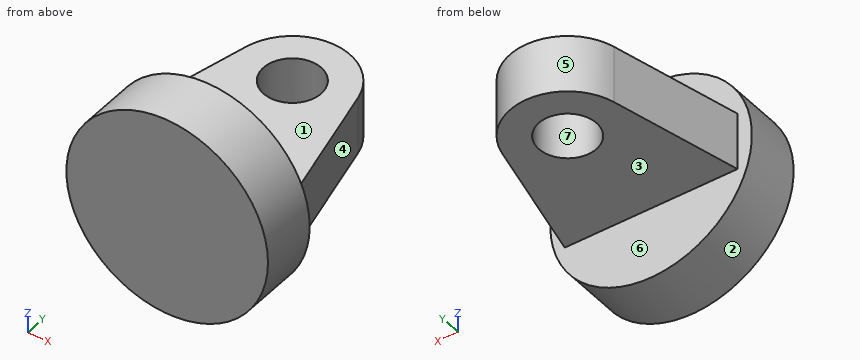
```python
from build123d import *

# Parameters (mm, degrees)
SKETCH_1_R           = 5
EXTRUDE_1_DEPTH      = 10
SKETCH_2_R           = 17.5
EXTRUDE_2_DEPTH      = 5
EXTRUDE_2_DEPTH_BACK = 5


with BuildPart() as part:
    # Sketch 1 → Extrude 1 (new body)
    with BuildSketch(Plane.XY):
        with BuildLine():
            Line((-5.269515354, 307.463167958), (-10.537394242, 285.164077124))
            Line((-10.537394242, 285.164077124), (-10.537394242, 280.164077124))
            Line((-10.537394242, 280.164077124), (19.462605758, 280.164077124))
            Line((19.462605758, 280.164077124), (19.462605758, 285.164077124))
            Line((19.462605758, 285.164077124), (14.19472687, 307.463167958))
            ThreePointArc((14.19472687, 307.463167958), (4.462605758, 315.164077124), (-5.269515354, 307.463167958))
        make_face()
        with Locations((4.462605758, 305.164077124)):
            Circle(SKETCH_1_R, mode=Mode.SUBTRACT)
    extrude(amount=EXTRUDE_1_DEPTH)

    # Sketch 2 → Extrude 2 (add, two sides)
    with BuildSketch(Plane.XZ.offset(-280.164077124)) as extrude_2_sk:
        with Locations((4.462605758, 5)):
            Circle(SKETCH_2_R)
    extrude(amount=EXTRUDE_2_DEPTH)
    extrude(extrude_2_sk.sketch, amount=-EXTRUDE_2_DEPTH_BACK)


solid = part.part
```
Build history of the part. All positions in model axes, mm. Face numbers are marked on the shaded views. A direction names the side the tool comes from. Give positions to 0.01 mm unless a question says otherwise; leave off trailing zeros. Loops run counter-clockwise (first coordinate to the right, second up) from the corner with the lowest first, then second, coordinate; pieces in that order, holes last. Notation, with made-up numbers: (28.5, 84.5) -> (86.5, 84.5) arc R12 cw to (86.5, 88.5) -> close; hole circle Ø3 at (30, 81.5). An arc over 180 degrees is marked (long way). One line per question, with ' | ' between items. Start each with the question number.
1) 3-axis set-ups, long thin cutter, end or side, ignore diameter. For the marked faces 1, 2 and 3: which of +Z, -Z, +X, -X, +Y, -Y reach the whole face in a straight line?
2) Cut at D-D (x = 13.5). Give the cut face in (y, z), plus the area to 3 significant figures.
3) Cut at A-A (y = 301.5). Give the cut face in (x, z), plus the area to 3 significant figures.
4) Probe L1, parallel to Z at x = 13.5, y = 298.5; L2, parallel to Y at x = -1, z = -9.5; L3, parallel to Y at x = 2.5, z = 9.5. List the from-to ranges inside material, lowest first.
5) Cut at B-B (z = 2.5). Give the cut face in (x, y).
6) Two-plate mould, pull along X, no slides. Class the marked faces 4, 5, 6 and 7: released by +X, released by -X, zero draft, split by the parting line, or undercut.
7) Pin check, flat tips, straight feed: pin 1 (1.5 mm diameter, centred on x = 14.5, y = 282.5, fed in from -Z); pin 2 (12 mm diameter, centred on y = 310, z = 11.5, fed in from +X); pin 3 (4 mm diameter, centred on x = 18.5, y = 291.5, fed in from -Z). Stop position of each tip, or through.
8) Cut at C-C (x = 6). Give the cut face in (y, z), plus the area to 3 significant figures.
Return value:
1) face 1: +Z, +X, -X, +Y | face 2: +Y, -Y | face 3: -Z, +X, -X, +Y
2) outline: (275.16, -9.99) -> (285.16, -9.99) -> (285.16, 0) -> (309.44, 0) -> (309.44, 10) -> (285.16, 10) -> (285.16, 19.99) -> (275.16, 19.99) -> close | area: 543 mm^2
3) outline: (-6.68, 0) -> (1.06, 0) -> (1.06, 10) -> (-6.68, 10) -> close; (7.86, 0) -> (15.6, 0) -> (15.6, 10) -> (7.86, 10) -> close | area: 155 mm^2
4) L1: 0 to 10 | L2: 275.16 to 285.16 | L3: 275.16 to 300.57, 309.76 to 314.97
5) outline: (-12.86, 275.16) -> (21.78, 275.16) -> (21.78, 285.16) -> (19.46, 285.16) -> (14.19, 307.46) arc R10 ccw to (-5.27, 307.46) -> (-10.54, 285.16) -> (-12.86, 285.16) -> close; hole circle Ø10 at (4.46, 305.16)
6) face 4: released by +X | face 5: split by the parting line | face 6: zero draft | face 7: undercut
7) pin 1: z = -9.83 | pin 2: x = 14.97 | pin 3: z = 0
8) outline: (275.16, -12.43) -> (285.16, -12.43) -> (285.16, 0) -> (300.41, 0) -> (300.41, 10) -> (285.16, 10) -> (285.16, 22.43) -> (275.16, 22.43) -> close; (309.92, 0) -> (315.05, 0) -> (315.05, 10) -> (309.92, 10) -> close | area: 552 mm^2
